```python
from build123d import *

# Parameters (mm, degrees)
SALIENTE_EXTRUIR1_DEPTH = 0.1


with BuildPart() as part:
    # Model → Saliente-Extruir1 (new body)
    with BuildSketch(Plane.XY):
        with BuildLine():
            Line((20.5, 22), (28.5, 22))
            Line((28.5, 22), (30.5, 22))
            ThreePointArc((30.5, 22), (32.621320344, 22.878679656), (33.5, 25))
            ThreePointArc((33.5, 25), (34.378679656, 27.121320344), (36.5, 28))
            ThreePointArc((36.5, 28), (38.621320344, 28.878679656), (39.5, 31))
            Line((39.5, 31), (39.5, 33))
            Line((39.5, 33), (39.5, 40))
            ThreePointArc((39.5, 40), (38.914213562, 41.414213562), (37.5, 42))
            Line((37.5, 42), (21.5, 42))
            ThreePointArc((21.5, 42), (20.085786438, 41.414213562), (19.5, 40))
            Line((19.5, 40), (19.5, 23))
            ThreePointArc((19.5, 23), (19.792893219, 22.292893219), (20.5, 22))
        make_face()
        with BuildLine():
            Line((31.5, 32), (33.156854249, 32))
            ThreePointArc((33.156854249, 32), (34.571067812, 32.585786438), (35.156854249, 34))
            Line((35.156854249, 34), (35.156854249, 35.656854249))
            ThreePointArc((35.156854249, 35.656854249), (34.571067812, 37.071067812), (33.156854249, 37.656854249))
            Line((33.156854249, 37.656854249), (25.843145751, 37.656854249))
            ThreePointArc((25.843145751, 37.656854249), (24.428932188, 37.071067812), (23.843145751, 35.656854249))
            Line((23.843145751, 35.656854249), (23.843145751, 28.343145751))
            ThreePointArc((23.843145751, 28.343145751), (24.428932188, 26.928932188), (25.843145751, 26.343145751))
            Line((25.843145751, 26.343145751), (27.5, 26.343145751))
            ThreePointArc((27.5, 26.343145751), (28.914213562, 26.928932188), (29.5, 28.343145751))
            Line((29.5, 28.343145751), (29.5, 30))
            ThreePointArc((29.5, 30), (30.085786438, 31.414213562), (31.5, 32))
        make_face(mode=Mode.SUBTRACT)
    extrude(amount=SALIENTE_EXTRUIR1_DEPTH)


solid = part.part
```
Verification items for the finished model (mm, model axes). Give positions to 0.01 mm unless a question says otherwise; leave off trailing zeros. Loops run counter-clockwise (first coordinate to the right, second up) from the corner with the lowest first, then second, coordinate; pieces in that order, holes last. Notation, with made-up numbers: M 34,10.25 L 73,10.25 A7 cw 73,21.25 Z; hole C 5.5,25 d2. An arc over 180 degrees is marked long. One line per question, with ' | ' between items.
Item 1: Section check B-B, the plane z = 0.05. Record the cut outline in (x, y).
Completed:
outline: M 19.5,23 A1 ccw 20.5,22 L 30.5,22 A3 ccw 33.5,25 A3 cw 36.5,28 A3 ccw 39.5,31 L 39.5,40 A2 ccw 37.5,42 L 21.5,42 A2 ccw 19.5,40 Z; hole M 23.84,28.34 A2 ccw 25.84,26.34 L 27.5,26.34 A2 ccw 29.5,28.34 L 29.5,30 A2 cw 31.5,32 L 33.16,32 A2 ccw 35.16,34 L 35.16,35.66 A2 ccw 33.16,37.66 L 25.84,37.66 A2 ccw 23.84,35.66 Z
Item 2: Section check D-D, the plane y = 23.5. Record the cut outline in (x, z).
Completed:
outline: M 19.5,0 L 33.1,0 L 33.1,0.1 L 19.5,0.1 Z
Item 3: Section check A-A, the plane x = 27.25. Record the cut outline in (y, z), plus the area to 3 significant figures.
Completed:
outline: M 22,0 L 26.34,0 L 26.34,0.1 L 22,0.1 Z; M 37.66,0 L 42,0 L 42,0.1 L 37.66,0.1 Z | area: 0.869 mm^2
Item 4: Section check C-C, the plane y = 36.25. Record the cut outline in (x, z).
Completed:
outline: M 19.5,0 L 23.93,0 L 23.93,0.1 L 19.5,0.1 Z; M 35.07,0 L 39.5,0 L 39.5,0.1 L 35.07,0.1 Z
Item 5: Thickness scan on line 1 (Y direction, x = 31.75, z = 0.05); line 2 (Y direction, x = 35.75, z = 0.05); line 3 (Y direction, x = 25, z = 0.05). Record the ranges inside material, lowest first. Write a range as [from, to].
Completed:
line 1: y = [22.27, 32], [37.66, 42] | line 2: y = [27.9, 42] | line 3: y = [22, 26.53], [37.47, 42]
